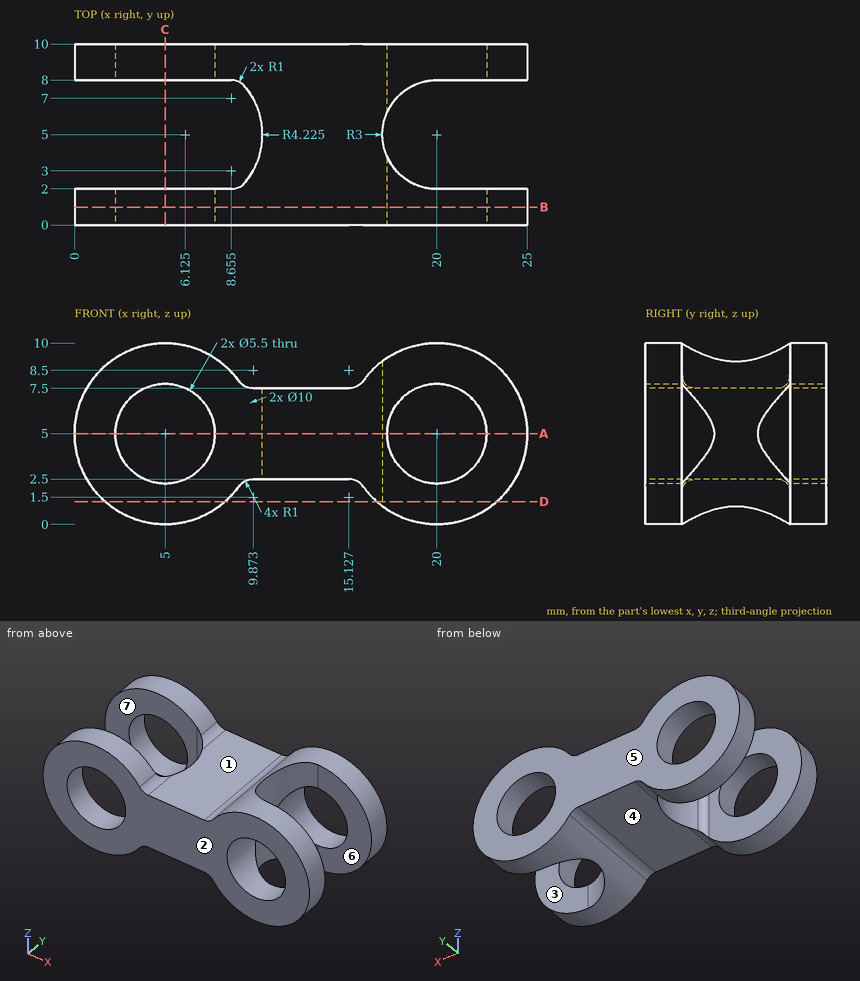
Answer from the drawing. Dimensions are ordinates in mm from the lowest x, y and z of the part. A direction names the side the tool comes from. Coordinates: 2 decimals unless noted, no trailing zeros. Loops run counter-clockwise (first coordinate to the right, second up) from the corner with the lowest first, then second, coordinate; pieces in that order, holes last. Notation, with made-up numbers: (68, 43.25) - (79, 43.25) arc R11 ccw to (79, 53.25) - close; hole circle Ø6 at (33.5, 22.5). An arc over 180 degrees is marked (long way). Use a Markdown table: item, result.
Item 1: For the marked faces 4, 5, 6 and 7, determine the directions among +Z, -Z, +X, -X, +Y, -Y from which every point of the face is accessible in a straight line to the end or side of a thin tool.
Evaluation:
| item | result |
|---|---|
| face 4 | -Z, +Y, -Y |
| face 5 | +Z, -Z, +X, -X, +Y |
| face 6 | +Z, -Z, +X |
| face 7 | +Z, -Z, -X |
Item 2: Find section C-C, the plane x = 5. Determine the outline of the cut face in (y, z), and give its area (3 significant figures).
Evaluation:
| item | result |
|---|---|
| outline | (0, 0) - (2, 0) - (2, 2.25) - (0, 2.25) - close; (0, 7.75) - (2, 7.75) - (2, 10) - (0, 10) - close; (8, 0) - (10, 0) - (10, 2.25) - (8, 2.25) - close; (8, 7.75) - (10, 7.75) - (10, 10) - (8, 10) - close |
| area | 18.0 mm2 |
Item 3: Find section D-D, the plane z = 1.25. Determine the outline of the cut face in (x, y).
Evaluation:
| item | result |
|---|---|
| outline | (1.69, 0) - (8.31, 0) - (8.31, 2) - (1.69, 2) - close; (1.69, 8) - (8.31, 8) - (8.31, 10) - (1.69, 10) - close; (16.69, 0) - (23.31, 0) - (23.31, 2) - (20, 2) arc R3 cw to (20, 8) - (23.31, 8) - (23.31, 10) - (16.69, 10) - close |
Item 4: Find section A-A, the plane z = 5. State how many separate pieces and enclosed holes the cut face has.
Evaluation:
| item | result |
|---|---|
| separate pieces | 5 |
| enclosed holes | 0 |
Item 5: The mould has two halves that part along Y. Classify the marked faces 1, 2 and 3: +Y half, -Y half, draft (parallel to the pull), parting line (faces both ways), or undercut.
Evaluation:
| item | result |
|---|---|
| face 1 | draft |
| face 2 | -Y half |
| face 3 | undercut |
Item 6: Find section B-B, the plane y = 1. Determine the outline of the cut face in (x, z), and give its area (3 significant figures).
Evaluation:
| item | result |
|---|---|
| outline | (9.06, 2.08) arc R1 cw to (9.87, 2.5) - (15.13, 2.5) arc R1 cw to (15.94, 2.08) arc R5 ccw (long way) to (15.94, 7.92) arc R1 cw to (15.13, 7.5) - (9.87, 7.5) arc R1 cw to (9.06, 7.92) arc R5 ccw (long way) to start; hole circle Ø5.5 at (5, 5); hole circle Ø5.5 at (20, 5) |
| area | 137 mm2 |
Item 7: Given pin 1 Ø3 at (y, z) = (5.5, 7.5) entering from +X (1 decimal); pin 2 Ø6 at (x, y) = (14, 6.5) entering from -Z; pin 3 Ø6 at (y, z) = (1, 9) entering from +X, each flat-ended and moving along its own axis, determine where each tip first touches the part or whether it passes through.
Evaluation:
| item | result |
|---|---|
| pin 1 | stops at x = 17.8 |
| pin 2 | stops at z = 1 |
| pin 3 | stops at x = 24.9 |
Item 8: Consider probe 1 along Y at (x, z) = (4.75, 8.5); probe 2 along X at (y, z) = (9.25, 6.5) (1 decimal); probe 3 along Y at (x, z) = (18, 8.25) (1 decimal). Determine where each line is inside the solid, lowest interval first. Write a range as from..to.
Evaluation:
| item | result |
|---|---|
| probe 1 | y = 0..2, 8..10 |
| probe 2 | x = 0.2..2.7, 7.3..17.7, 22.3..24.8 |
| probe 3 | y = 0..2.8, 7.2..10 |
